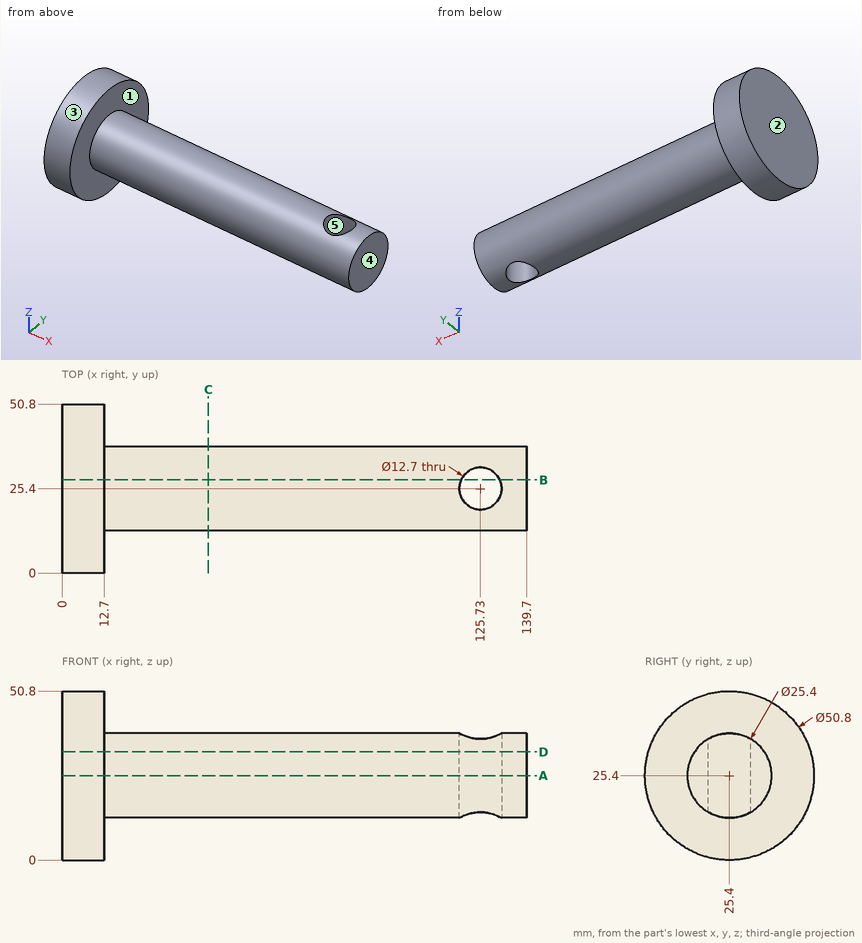
Geometry check sheet. Reference: drawing and pictorial views, mm from the part's lowest x, y, z. A direction names the side the tool comes from. Round coordinates to 2 decimals unless told otherwise and drop trailing zeros. Write each loop counter-clockwise with the first axis right and the second up, starting at its lowest first coordinate (ties: lowest second). Pieces come first, ordered by that corner, then holes. Notation, with made-up numbers: (-21.75, 71) -> (-17.75, 71) arc R14 ccw to (-17.75, 80) -> close; hole circle Ø6 at (-3.75, -35.5). An arc over 180 degrees is marked (long way). Answer as CSV lines item,"result". Start each with the question number.
1) Tool access check on the marked faces 1 and 2. Record the directions out of +Z, -Z, +X, -X, +Y, -Y that give a thin tool (end or side, any length) a straight path to the whole face; none if there is none.
2) Section check B-B on y = 28. Enter the section's corners in (x, z), and give its area (3 significant figures).
3) Release check for a two-part mould opening along X. For the marked faces 3, 4 and 5 record: pulls with the +X half, pulls with the -X half, needs draft (parallel to the pull), parting line crosses it, or undercut.
4) Go/stop test with flat-tipped pins: P1, Ø10, axis at x = 59.5, y = 37, coming from the +Z side; P2, Ø4, axis at x = 48, z = 26, coming from the +Y side; P3, Ø1.5, axis at x = 82, z = 19, coming from the -Y side; P4, Ø11.5, axis at x = 125.73, y = 25.4, coming from the -Z side. Record where each tip stops, or that it passes through.
5) Section check C-C on x = 44. Enter the section's corners in (y, z), and give its area (3 significant figures).
6) Material ranges on line 1 (X direction, y = 25, z = 33); line 2 (X direction, y = 36, z = 4); line 3 (Y direction, x = 125, z = 30), recorded low to high. Write a range as from..to.
7) Section check A-A on z = 25.4. Enter the section's corners in (x, y), and give its area (3 significant figures).
8) Section check D-D on z = 32.5. Enter the section's corners in (x, y), and give its area (3 significant figures).
Found:
1,face 1,"+X"
1,face 2,"+Z, -Z, -X, +Y, -Y"
2,outline,"(0, 0.13) -> (12.7, 0.13) -> (12.7, 12.97) -> (119.94, 12.97) -> (119.94, 37.83) -> (12.7, 37.83) -> (12.7, 50.67) -> (0, 50.67) -> close; (131.52, 12.97) -> (139.7, 12.97) -> (139.7, 37.83) -> (131.52, 37.83) -> close"
2,area,"3,510 mm^2"
3,face 3,"needs draft"
3,face 4,"pulls with the +X half"
3,face 5,"undercut"
4,P1,"stops at z = 36.25"
4,P2,"stops at y = 38.1"
4,P3,"stops at y = 14.03"
4,P4,"passes through"
5,outline,"circle Ø25.4 at (25.4, 25.4)"
5,area,"507 mm^2"
6,line 1,"x = 0..119.39, 132.07..139.7"
6,line 2,"x = 0..12.7"
6,line 3,"y = 13.56..19.09, 31.71..37.24"
7,outline,"(0, 0) -> (12.7, 0) -> (12.7, 12.7) -> (139.7, 12.7) -> (139.7, 38.1) -> (12.7, 38.1) -> (12.7, 50.8) -> (0, 50.8) -> close; hole circle Ø12.7 at (125.73, 25.4)"
7,area,"3,740 mm^2"
8,outline,"(0, 1.01) -> (12.7, 1.01) -> (12.7, 14.87) -> (139.7, 14.87) -> (139.7, 35.93) -> (12.7, 35.93) -> (12.7, 49.79) -> (0, 49.79) -> close; hole circle Ø12.7 at (125.73, 25.4)"
8,area,"3,170 mm^2"
